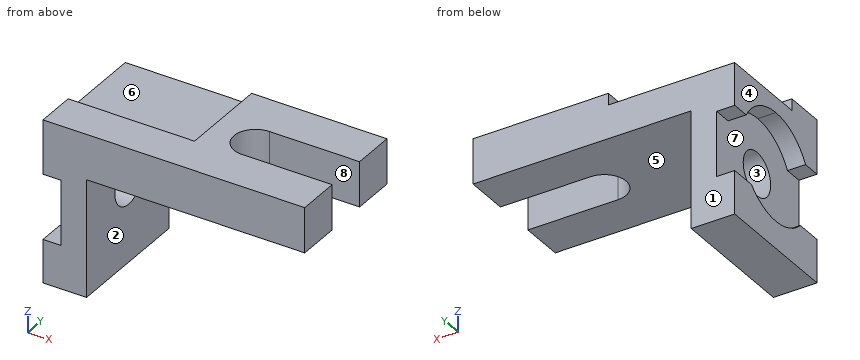
from build123d import *

# Parameters (mm, degrees)
SKETCH1_W               = 145
SKETCH1_H               = 72
BOSS_EXTRUDE1_DEPTH     = 25
BOSS_EXTRUDE13_DEPTH    = 72
SKETCH16_R              = 12
CUT_EXTRUDE1_DEPTH      = 10
CUT_EXTRUDE2_DEPTH      = 175.453432182
CUT_EXTRUDE2_DEPTH_BACK = 50
SKETCH17_W              = 70
SKETCH17_H              = 6.390151493
SKETCH18_R              = 12
CUT_EXTRUDE3_DEPTH      = 24
CUT_EXTRUDE4_DEPTH      = 175.453432182
CUT_EXTRUDE4_DEPTH_BACK = 25


with BuildPart() as part:
    # Sketch1 → Boss-Extrude1 (new body)
    with BuildSketch(Plane.XY):
        with Locations((72.5, 36)):
            Rectangle(SKETCH1_W, SKETCH1_H)
    extrude(amount=BOSS_EXTRUDE1_DEPTH)

    # Sketch5 → Boss-Extrude13 (add)
    with BuildSketch(Plane(origin=(0, 72, 0), x_dir=(1, 0, 0), z_dir=(0, 1, 0))):
        Polygon((0, 65), (0, 0), (1.798699266, 0), (24.115506302, 0), (24.115506302, 65), align=None)
    extrude(amount=-BOSS_EXTRUDE13_DEPTH)

    # Sketch16 → Cut-Extrude1 (cut)
    # profile 1 of 6: a face of its own
    with BuildSketch(Plane.ZY):
        with BuildLine():
            ThreePointArc((-5, 61.980762114), (-23.767010787, 65.762554153), (-41, 57.424285286))
            Line((-41, 57.424285286), (-41, 14.575714714))
            ThreePointArc((-41, 14.575714714), (-23.767010787, 6.237445847), (-5, 10.019237886))
            Line((-5, 10.019237886), (-5, 61.980762114))
        make_face()
        with Locations((-20, 36)):
            Circle(SKETCH16_R, mode=Mode.SUBTRACT)
    # profile 2 of 6: a face of its own
    with BuildSketch(Plane.ZY):
        with Locations((-20, 36)):
            Circle(SKETCH16_R)
    # profile 3 of 6: a face of its own
    with BuildSketch(Plane.ZY):
        with BuildLine():
            ThreePointArc((10, 36), (5.980762114, 51), (-5, 61.980762114))
            Line((-5, 61.980762114), (-5, 10.019237886))
            ThreePointArc((-5, 10.019237886), (5.980762114, 21), (10, 36))
        make_face()
    # profile 4 of 6: a face of its own
    with BuildSketch(Plane.ZY):
        with BuildLine():
            Line((-41, 14.575714714), (-41, 57.424285286))
            ThreePointArc((-41, 57.424285286), (-50, 36), (-41, 14.575714714))
        make_face()
    # profile 5 of 6: a face of its own
    with BuildSketch(Plane.ZY):
        with BuildLine():
            Line((-5, 72), (-41, 72))
            Line((-41, 72), (-41, 57.424285286))
            ThreePointArc((-41, 57.424285286), (-23.767010787, 65.762554153), (-5, 61.980762114))
            Line((-5, 61.980762114), (-5, 72))
        make_face()
    # profile 6 of 6: a face of its own
    with BuildSketch(Plane.ZY):
        with BuildLine():
            ThreePointArc((-5, 10.019237886), (-23.767010787, 6.237445847), (-41, 14.575714714))
            Line((-41, 14.575714714), (-41, 0))
            Line((-41, 0), (-5, 0))
            Line((-5, 0), (-5, 10.019237886))
        make_face()
    extrude(amount=-CUT_EXTRUDE1_DEPTH, mode=Mode.SUBTRACT)

    # Sketch17 → Cut-Extrude2 (cut, two sides: drawn at the far end of the back side and taken through both)
    with BuildSketch(Plane(origin=(0, 72, 0), x_dir=(1, 0, 0), z_dir=(0, 1, 0)).offset(-CUT_EXTRUDE2_DEPTH_BACK)):
        with Locations((35, -21.804924254)):
            Rectangle(SKETCH17_W, SKETCH17_H)
    extrude(amount=CUT_EXTRUDE2_DEPTH + CUT_EXTRUDE2_DEPTH_BACK, mode=Mode.SUBTRACT)

    # Sketch18 → Cut-Extrude3 (cut)
    with BuildSketch(Plane.ZY.offset(-10)):
        with Locations((-20.942172697, 36.785143914)):
            Circle(SKETCH18_R)
    extrude(amount=-CUT_EXTRUDE3_DEPTH, mode=Mode.SUBTRACT)

    # Sketch19 → Cut-Extrude4 (cut, two sides: drawn at the far end of the back side and taken through both)
    with BuildSketch(Plane(origin=(0, 0, 0), x_dir=(-1, 0, 0), z_dir=(0, 0, -1)).offset(-CUT_EXTRUDE4_DEPTH_BACK)):
        with BuildLine():
            Line((-145, 24), (-95, 24))
            ThreePointArc((-95, 24), (-83, 36), (-95, 48))
            Line((-95, 48), (-145, 48))
            Line((-145, 48), (-145, 24))
        make_face()
    extrude(amount=CUT_EXTRUDE4_DEPTH + CUT_EXTRUDE4_DEPTH_BACK, mode=Mode.SUBTRACT)


solid = part.part
Geometry check sheet. Reference: the model listing, model coordinates, mm. Face numbers are marked on the shaded views. A direction names the side the tool comes from. Round coordinates to 2 decimals unless told otherwise and drop trailing zeros. Order: outer loops, then holes, each group sorted by start corner. A loop starts at its lowest first (then second) coordinate and runs counter-clockwise, first axis right, second up. Notation, with made-up numbers: M 10,1 L 63,1 A11 cw 63,22 Z; hole C 36,-29.5 d7. An arc over 180 degrees is marked long. Answer in a Markdown table with one row per item.
(1) Sectioned sample at B-B, the plane y = 60. Record the cut outline in (x, z).
Responses:
| item | result |
|---|---|
| outline | M 0,-65 L 24.12,-65 L 24.12,0 L 145,0 L 145,25 L 70,25 L 70,18.61 L 0,18.61 L 0,-2 L 10,-2 L 10,-41 L 0,-41 Z |
(2) Sectioned sample at A-A, the plane x = 104. Record the cut outline in (y, z), and give its area (3 significant figures).
Responses:
| item | result |
|---|---|
| outline | M 0,0 L 24,0 L 24,25 L 0,25 Z; M 48,0 L 72,0 L 72,25 L 48,25 Z |
| area | 1,200 mm² |
(3) Tool access check on the marked faces 4, 5, 6, 7 and 8. Record the directions out of +Z, -Z, +X, -X, +Y, -Y that give a thin tool (end or side, any length) a straight path to the whole face; none if there is none.
Responses:
| item | result |
|---|---|
| face 4 | +Z, -Z, -X, +Y, -Y |
| face 5 | -Z, +X, +Y, -Y |
| face 6 | +Z, -X, +Y |
| face 7 | -X |
| face 8 | +Z, -Z, +X |
(4) Sectioned sample at C-C, the plane y = 32.5. Record the cut outline in (x, z), and give its area (3 significant figures).
Responses:
| item | result |
|---|---|
| outline | M 0,-65 L 24.12,-65 L 24.12,-32.15 L 10,-32.15 L 10,-49.8 L 0,-49.8 Z; M 0,9.8 L 10,9.8 L 10,-9.73 L 24.12,-9.73 L 24.12,0 L 83.52,0 L 83.52,25 L 70,25 L 70,18.61 L 0,18.61 Z |
| area | 2,300 mm² |
(5) Scan lines: probe 1 along X at (y, z) = (17.5, -35); probe 2 along Z at (x, y) = (77.5, 11); probe 3 along Y at (x, z) = (106.5, 17). Record each from-to range of solid material in increasing order. Write a range as from..to.
Responses:
| item | result |
|---|---|
| probe 1 | x = 10..24.12 |
| probe 2 | z = 0..25 |
| probe 3 | y = 0..24, 48..72 |
(6) Sectioned sample at D-D, the plane z = -22.5. Record the cut outline in (x, y).
Responses:
| item | result |
|---|---|
| outline | M 10,0 L 24.12,0 L 24.12,24.89 L 10,24.89 Z; M 10,48.68 L 24.12,48.68 L 24.12,72 L 10,72 Z |
(7) Go/stop test with flat-tipped pins: P1, Ø25, axis at x = 41, y = 54.5, coming from the +Z side; P2, Ø1, axis at y = 24.5, z = -12, coming from the +X side; P3, Ø5, axis at x = 50, z = 23.5, coming from the +Y side; P4, Ø1, axis at x = 87, y = 44, coming from the +Z side. Record where each tip stops, or that it passes through.
Responses:
| item | result |
|---|---|
| P1 | stops at z = 18.61 |
| P2 | stops at x = 24.12 |
| P3 | stops at y = 22 |
| P4 | passes through |
(8) Draft check along Y on the marked faces 1, 2 and 3. Enter one of: released by +Y, released by -Y, zero draft, split by the parting line, or undercut.
Responses:
| item | result |
|---|---|
| face 1 | released by +Y |
| face 2 | zero draft |
| face 3 | undercut |
